```python
from build123d import *

# Parameters (mm, degrees)
ESBO_O1_R             = 57.5
ESBO_O1_R_2           = 7.5
EXTRUS_O1_DEPTH       = 10
EXTRUS_O2_DEPTH       = 3
ESBO_O3_W             = 5
ESBO_O3_H             = 9.7
CORTE_EXTRUS_O1_DEPTH = 82.929848041


with BuildPart() as part:
    # Esboço1 → Extrusão1 (new body)
    with BuildSketch(Plane.XY):
        Circle(ESBO_O1_R)
        Circle(ESBO_O1_R_2, mode=Mode.SUBTRACT)
    extrude(amount=-EXTRUS_O1_DEPTH)

    # Esboço2 → Extrusão2 (add)
    with BuildSketch(Plane.XY):
        with BuildLine():
            Line((5, 54.270157545), (5, 21.937410968))
            ThreePointArc((5, 21.937410968), (17.589059099, 14.0312152), (22.5, 0))
            ThreePointArc((22.5, 0), (22.248179609, -3.35685926), (21.498355192, -6.638578465))
            Line((21.498355192, -6.638578465), (49.499335102, -22.804951754))
            ThreePointArc((49.499335102, -22.804951754), (53.235156443, -11.673393615), (54.5, 0))
            ThreePointArc((54.5, 0), (40.266301047, 36.72703364), (5, 54.270157545))
        make_face()
        with BuildLine():
            ThreePointArc((-21.498355192, -6.638578465), (-19.485571585, 11.25), (-5, 21.937410968))
            Line((-5, 21.937410968), (-5, 54.270157545))
            ThreePointArc((-5, 54.270157545), (-47.198384506, 27.25), (-49.499335102, -22.804951754))
            Line((-49.499335102, -22.804951754), (-21.498355192, -6.638578465))
        make_face()
        with BuildLine():
            Line((44.499335102, -31.465205792), (16.498355192, -15.298832503))
            ThreePointArc((16.498355192, -15.298832503), (0, -22.5), (-16.498355192, -15.298832503))
            Line((-16.498355192, -15.298832503), (-44.499335102, -31.465205792))
            ThreePointArc((-44.499335102, -31.465205792), (0, -54.5), (44.499335102, -31.465205792))
        make_face()
    extrude(amount=EXTRUS_O2_DEPTH)

    # Esboço3 → Corte-extrusão1 (cut, through all)
    with BuildSketch(Plane.XY):
        with Locations((0, 4.85)):
            Rectangle(ESBO_O3_W, ESBO_O3_H)
    extrude(amount=-CORTE_EXTRUS_O1_DEPTH, mode=Mode.SUBTRACT)


solid = part.part
```
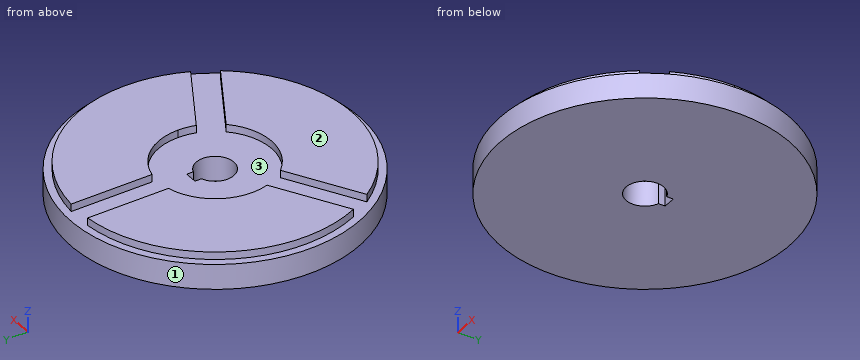
Verification items for the finished model (mm, model axes). Face numbers are marked on the shaded views. Coordinates: 2 decimals unless noted, no trailing zeros. Write each loop counter-clockwise with the first axis right and the second up, starting at its lowest first coordinate (ties: lowest second). Pieces come first, ordered by that corner, then holes. Notation, with made-up numbers: (62, 32.5) - (79, 32.5) arc R10 ccw to (79, 47.5) - close; hole circle Ø9 at (23.25, 67.25). An arc over 180 degrees is marked (long way). Write item = value, one per line.
Q1. Cross-section at B-B (z = -4.25). Enter the section's corners in (x, y), plus the area to 3 significant figures.
Answer:
outline = circle Ø115 at (0, 0); hole (-2.5, 7.07) arc R7.5 ccw (long way) to (2.5, 7.07) - (2.5, 9.7) - (-2.5, 9.7) - close
area = 10,200 mm²
Q2. Go/stop test with flat-tipped pins: pin 1 Ø0.8 at (y, z) = (8, -7) entering from +X; pin 2 Ø1 at (x, z) = (-20.5, -6.5) entering from -Y; pin 3 Ø1.5 at (x, z) = (0.5, -5) entering from +Y. Record where each tip stops, or that it passes through.
Answer:
pin_1 = 57
pin_2 = -53.91
pin_3 = 57.5
Q3. Cross-section at C-C (y = 5). Enter the section's corners in (x, z), plus the area to 3 significant figures.
Answer:
outline = (-57.28, -10) - (-5.59, -10) - (-5.59, 0) - (-21.94, 0) - (-21.94, 3) - (-54.27, 3) - (-54.27, 0) - (-57.28, 0) - close; (5.59, -10) - (57.28, -10) - (57.28, 0) - (54.27, 0) - (54.27, 3) - (21.94, 3) - (21.94, 0) - (5.59, 0) - close
area = 1,230 mm²
Q4. Cross-section at D-D (y = -9). Enter the section's corners in (x, z), plus the area to 3 significant figures.
Answer:
outline = (-56.79, -10) - (56.79, -10) - (56.79, 0) - (53.75, 0) - (53.75, 3) - (25.59, 3) - (25.59, 0) - (-25.59, 0) - (-25.59, 3) - (-53.75, 3) - (-53.75, 0) - (-56.79, 0) - close
area = 1,300 mm²
Q5. Mould release check, pull along Y, two halves, no side actions. Record for the marked faces 1, 2 and 3: released by +Y, released by -Y, zero draft, split by the parting line, or undercut.
Answer:
face_1 = split by the parting line
face_2 = zero draft
face_3 = undercut
Q6. Cross-section at A-A (x = 0). Enter the section's corners in (y, z), plus the area to 3 significant figures.
Answer:
outline = (-57.5, -10) - (-7.5, -10) - (-7.5, 0) - (-22.5, 0) - (-22.5, 3) - (-54.5, 3) - (-54.5, 0) - (-57.5, 0) - close; (9.7, -10) - (57.5, -10) - (57.5, 0) - (9.7, 0) - close
area = 1,070 mm²
Q7. Material ranges on L1, parallel to Y at x = 0, z = -5; L2, parallel to X at y = 13.5, z = 1.5; L3, parallel to X at y = 25, z = 1, recorded low to high. Write a range as from..to.
Answer:
L1 = -57.5..-7.5, 9.7..57.5
L2 = -52.8..-18, 18..52.8
L3 = -48.43..-5, 5..48.43
